from build123d import *

# Parameters (mm, degrees)
F0_R     = 28.575
F1_DEPTH = 40.2336
F2_R     = 10.16
F3_DEPTH = 15.7734
F4_DEPTH = 25.4
F5_R     = 3.302


with BuildPart() as f1:
    # F0 (on Top) → F1 (new body)
    with BuildSketch(Plane.XY):
        Circle(F0_R)
        with BuildLine():
            ThreePointArc((-13.4477648793, -4.826), (-14.2875, 0), (-13.4477648793, 4.826))
            ThreePointArc((-13.4477648793, 4.826), (0, 14.2875), (13.4477648793, 4.826))
            Line((13.4477648793, 4.826), (16.8290351207, 4.826))
            Line((16.8290351207, 4.826), (16.8290351207, -4.826))
            Line((16.8290351207, -4.826), (13.4477648793, -4.826))
            ThreePointArc((13.4477648793, -4.826), (0, -14.2875), (-13.4477648793, -4.826))
        make_face(mode=Mode.SUBTRACT)
    extrude(amount=F1_DEPTH)

    # F2 (on Top) → F3 (join)
    with BuildSketch(Plane.XY):
        with BuildLine():
            ThreePointArc((57.1919272622, -18.7764181619), (34.925, 0), (57.1919272622, 18.7764181619))
            Line((57.1919272622, 18.7764181619), (9.5121844836, 26.9452959039))
            ThreePointArc((9.5121844836, 26.9452959039), (23.3274655355, 16.5033322905), (28.575, 0))
            ThreePointArc((28.575, 0), (23.3274655355, -16.5033322905), (9.5121844836, -26.9452959039))
            Line((9.5121844836, -26.9452959039), (57.1919272622, -18.7764181619))
        make_face()
        with BuildLine():
            ThreePointArc((57.1919272622, -18.7764181619), (68.5383952831, -12.2804730295), (73.025, 0))
            ThreePointArc((73.025, 0), (68.5383952831, 12.2804730295), (57.1919272622, 18.7764181619))
            ThreePointArc((57.1919272622, 18.7764181619), (34.925, 0), (57.1919272622, -18.7764181619))
        make_face()
        with Locations((53.975, 0)):
            Circle(F2_R, mode=Mode.SUBTRACT)
    extrude(amount=F3_DEPTH)

    # F0 (on Top) → F4 (join)
    with BuildSketch(Plane.XY):
        Circle(F0_R)
        with BuildLine():
            ThreePointArc((-13.4477648793, -4.826), (-14.2875, 0), (-13.4477648793, 4.826))
            ThreePointArc((-13.4477648793, 4.826), (0, 14.2875), (13.4477648793, 4.826))
            Line((13.4477648793, 4.826), (16.8290351207, 4.826))
            Line((16.8290351207, 4.826), (16.8290351207, -4.826))
            Line((16.8290351207, -4.826), (13.4477648793, -4.826))
            ThreePointArc((13.4477648793, -4.826), (0, -14.2875), (-13.4477648793, -4.826))
        make_face(mode=Mode.SUBTRACT)
    extrude(amount=F4_DEPTH)

    # F5
    f5_edges = [f1.edges().sort_by_distance(p)[0] for p in [
        (-28.575, 0, 40.2336),
    ]]
    fillet(f5_edges, radius=F5_R)


solid = f1.part
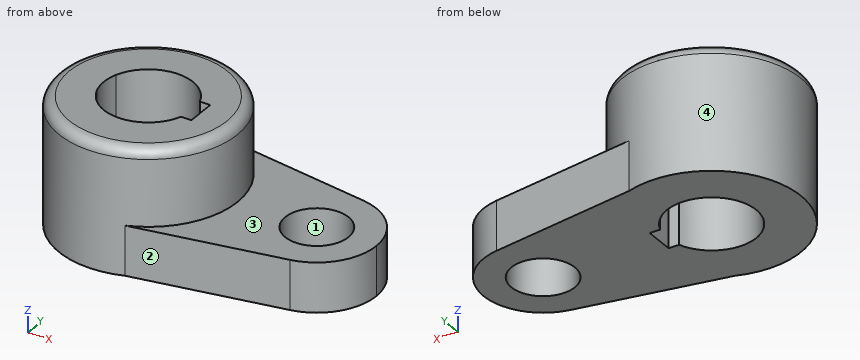
CAD build for the part. Positions are in the model's coordinates, mm. Face numbers are marked on the shaded views. Round coordinates to 2 decimals unless told otherwise and drop trailing zeros. Order: outer loops, then holes, each group sorted by start corner. A loop starts at its lowest first (then second) coordinate and runs counter-clockwise, first axis right, second up. Notation, with made-up numbers: (-23.5, -23) -> (13.5, -23) arc R14 cw to (13.5, -19) -> close; hole circle Ø4 at (-10.5, 83.25). An arc over 180 degrees is marked (long way). Write each question's results on one line, items separated by ' | '.
1. Cut at A-A (z = 14.5). Count the separate pieces of the cut face and the enclosed holes in it, plus the area to 3 significant figures.
Findings below:
separate pieces: 1 | enclosed holes: 2 | area: 3,450 mm²
2. Pull direction X, two halves, no side cores. Call the marked faces 1, 2, 3 and 4: pulls with the +X half, pulls with the -X half, needs draft (parallel to the pull), parting line crosses it, or undercut.
Findings below:
face 1: undercut | face 2: pulls with the +X half | face 3: needs draft | face 4: parting line crosses it
3. Flat gauge pins, fed straight in: P1, Ø5, axis at x = 15, z = 7, coming from the -Y side; P2, Ø1, axis at x = 15.5, z = 28, coming from the -Y side; P3, Ø1, axis at x = 62.5, y = 17.5, coming from the +Z side; P4, Ø5, axis at y = 2, z = 29.5, coming from the -X side (3 decimals). Where does each tip first touch, or does it go through?
Findings below:
P1: stops at y = -26.43 | P2: stops at y = -24.32 | P3: stops at z = 15.77 | P4: stops at x = -28.575
4. Wall check: line 1 along Y through (x, z) = (-10, 5); line 2 along Z through (x, y) = (31, 19.5); line 3 along X through (y, z) = (2.5, 34.5). Give the ranges that are in metal, low to high. Write a range as [from, to].
Findings below:
line 1: y = [-26.77, -10.2], [10.2, 26.77] | line 2: z = [0, 15.77] | line 3: x = [-28.47, -14.07], [16.83, 28.47]
5. Cut at B-B (x = 0). Give the cut face in (y, z) (1 decimal), plus the area to 3 significant figures.
Findings below:
outline: (-28.6, 0) -> (-14.3, 0) -> (-14.3, 40.2) -> (-25.3, 40.2) arc R3.3 ccw to (-28.6, 36.9) -> close; (14.3, 0) -> (28.6, 0) -> (28.6, 36.9) arc R3.3 ccw to (25.3, 40.2) -> (14.3, 40.2) -> close | area: 1,140 mm²
